Geometry: final body of the model. Coordinates: model frame, mm. A direction names the side the tool comes from. Give positions to 0.01 mm unless a question says otherwise; leave off trailing zeros. Order: outer loops, then holes, each group sorted by start corner. A loop starts at its lowest first (then second) coordinate and runs counter-clockwise, first axis right, second up. Notation, with made-up numbers: (7, -24.75) -> (18, -24.75) arc R27 ccw to (18, 13.25) -> close; hole circle Ø8 at (59.25, 10.5). An arc over 180 degrees is marked (long way). Write item = value, one per line.
```python
from build123d import *

# Parameters (mm, degrees)
F0_R     = 8.75
F0_R_2   = 7
F1_DEPTH = 40
F2_DEPTH = 20


with BuildPart() as f1:
    # F0 (on Front) → F1 (new body)
    with BuildSketch(Plane.XZ):
        with BuildLine():
            ThreePointArc((-2.728431, 10.65625), (-6.744897, -8.68944), (11, 0))
            ThreePointArc((11, 0), (8.68944, 6.744897), (2.728431, 10.65625))
            ThreePointArc((2.728431, 10.65625), (0, 10), (-2.728431, 10.65625))
        make_face()
        Circle(F0_R, mode=Mode.SUBTRACT)
        Circle(F0_R)
        Circle(F0_R_2, mode=Mode.SUBTRACT)
    extrude(amount=F1_DEPTH)

    # F0 (on Front) → F2 (cut)
    with BuildSketch(Plane.XZ):
        Circle(F0_R)
        Circle(F0_R_2, mode=Mode.SUBTRACT)
    extrude(amount=F2_DEPTH, mode=Mode.SUBTRACT)


solid = f1.part
```
1) Mould query, pull axis X, two halves, no side actions, for faces 3 (the face through (7.2, -40, 0)), 4 (the face through (6.466, -29.86, -2.681)). Classes: +X half, -X half, draft (parallel to the pull), parting line (faces both ways), or undercut.
Check sheet entries:
face_3 = draft
face_4 = undercut
2) First-contact query: P1, Ø6, axis at y = -13, z = -8, coming from the -X side; P2, Ø1.5, axis at x = -1, z = -5.5, coming from the -Y side (3 decimals); P3, Ø3, axis at y = -24.5, z = 5, coming from the +X side. Flat tips, straight axial feed; report the tip coordinate or a pass-through.
Check sheet entries:
P1 = -9.8
P2 = through
P3 = 10.43
3) Section query C-C (y = -26). Output: boundary loops of the cut face in (x, z).
Check sheet entries:
outline = (-2.73, 10.66) arc R11 ccw (long way) to (2.73, 10.66) arc R6 cw to start; hole circle Ø14 at (0, 0)
4) Line query: line 1 (X direction, y = -22.5, z = 5.5); line 2 (Z direction, x = -1.25, y = -22); line 3 (Z direction, x = -3, y = -26). Output: solid intervals per line, ascending. Write a range as from..to.
Check sheet entries:
line_1 = -9.53..-4.33, 4.33..9.53
line_2 = -10.93..-6.89, 6.89..10.13
line_3 = -10.58..-6.32, 6.32..10.58
5) Section query D-D (y = -14.5). Output: boundary loops of the cut face in (x, z).
Check sheet entries:
outline = (-2.73, 10.66) arc R11 ccw (long way) to (2.73, 10.66) arc R6 cw to start; hole circle Ø17.5 at (0, 0)
6) Section query A-A (x = 0). Output: boundary loops of the cut face in (y, z), plus the area to 3 significant figures.
Check sheet entries:
outline = (-40, -11) -> (0, -11) -> (0, -8.75) -> (-20, -8.75) -> (-20, -7) -> (-40, -7) -> close; (-40, 7) -> (-20, 7) -> (-20, 8.75) -> (0, 8.75) -> (0, 10) -> (-40, 10) -> close
area = 210 mm²
7) Section query B-B (z = 2). Output: boundary loops of the cut face in (x, y).
Check sheet entries:
outline = (-10.82, -40) -> (-6.71, -40) -> (-6.71, -20) -> (-8.52, -20) -> (-8.52, 0) -> (-10.82, 0) -> close; (6.71, -40) -> (10.82, -40) -> (10.82, 0) -> (8.52, 0) -> (8.52, -20) -> (6.71, -20) -> close
8) Reachability of faces 1 (the face through (-6.944, -9.86, -5.324)), 2 (the face through (-1, 0, -9)) from +Z, -Z, +X, -X, +Y, -Y: full face, straight path, thin tool, end or side. Return the list, or none.
Check sheet entries:
face_1 = +Y
face_2 = +Z, -Z, +X, -X, +Y
